CAD build for the part. Positions are in the model's coordinates, mm. Face numbers are marked on the shaded views. A direction names the side the tool comes from. Round coordinates to 2 decimals unless told otherwise and drop trailing zeros. Loops run counter-clockwise (first coordinate to the right, second up) from the corner with the lowest first, then second, coordinate; pieces in that order, holes last. Notation, with made-up numbers: (21.5, -18.5) - (62.5, -18.5) arc R28 ccw to (62.5, 0.5) - close; hole circle Ø11 at (60.25, -15.5). An arc over 180 degrees is marked (long way). One line per question, with ' | ' between items.
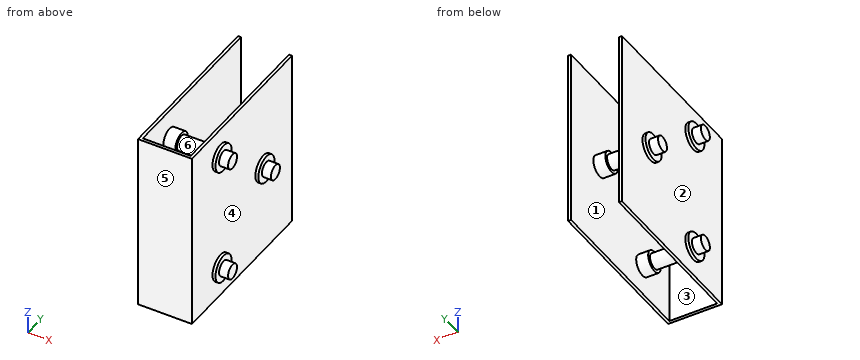
```python
from build123d import *

# Parameters (mm, degrees)
BOSS_EXTRUDE1_DEPTH      = 95.25
BOSS_EXTRUDE2_DEPTH      = 1.5875
BOSS_EXTRUDE2_DEPTH_BACK = 30.1625
SKETCH3_R                = 5.55625
SKETCH4_R                = 7.14375
BOSS_EXTRUDE3_DEPTH      = 1.5875
BOSS_EXTRUDE4_START      = 1.5875
SKETCH5_R                = 7.14375
BOSS_EXTRUDE4_DEPTH      = 1.5875
SKETCH7_W                = 12.7
SKETCH7_H                = 95.25
CUT_EXTRUDE1_DEPTH       = 131.184679518
BOSS_EXTRUDE5_DEPTH      = 6.35
BOSS_EXTRUDE5_DEPTH_BACK = 34.9377
SKETCH6_R                = 3.96875


with BuildPart() as part:
    # Sketch1 → Boss-Extrude1 (new body)
    with BuildSketch(Plane.XY):
        Polygon((-14.2875, 88.9), (-14.2875, 0), (14.2875, 0), (14.2875, 88.9), (12.7, 88.9), (12.7, 1.5875), (-12.7, 1.5875), (-12.7, 88.9), align=None)
    extrude(amount=BOSS_EXTRUDE1_DEPTH)

    # Sketch3 → Boss-Extrude2 (add, two sides: drawn at the far end of the back side and taken through both)
    with BuildSketch(Plane(origin=(14.2875, 0, 0), x_dir=(0, 0, -1), z_dir=(1, 0, 0)).offset(-BOSS_EXTRUDE2_DEPTH_BACK)):
        with Locations(Location((-47.625, 63.5, 0), (0, 0, 90))):
            Circle(SKETCH3_R)
        with Locations(Location((-79.375, 25.4, 0), (0, 0, 90))):
            Circle(SKETCH3_R)
        with Locations(Location((-15.875, 25.4, 0), (0, 0, 90))):
            Circle(SKETCH3_R)
    extrude(amount=BOSS_EXTRUDE2_DEPTH + BOSS_EXTRUDE2_DEPTH_BACK)

    # Sketch4 → Boss-Extrude3 (add)
    with BuildSketch(Plane(origin=(14.2875, 0, 0), x_dir=(0, 0, -1), z_dir=(1, 0, 0))):
        with Locations(Location((-47.625, 63.5, 0), (0, 0, 270))):
            Circle(SKETCH4_R)
        with Locations(Location((-15.875, 25.4, 0), (0, 0, 270))):
            Circle(SKETCH4_R)
        with Locations(Location((-79.375, 25.4, 0), (0, 0, 270))):
            Circle(SKETCH4_R)
    extrude(amount=BOSS_EXTRUDE3_DEPTH)

    # Sketch5 → Boss-Extrude4 (add)
    with BuildSketch(Plane.ZY.offset(14.2875).offset(BOSS_EXTRUDE4_START)):
        with Locations(Location((47.625, 63.5, 0), (0, 0, 270))):
            Circle(SKETCH5_R)
        with Locations(Location((79.375, 25.4, 0), (0, 0, 270))):
            Circle(SKETCH5_R)
        with Locations(Location((15.875, 25.4, 0), (0, 0, 270))):
            Circle(SKETCH5_R)
    extrude(amount=-BOSS_EXTRUDE4_DEPTH)

    # Sketch7 → Cut-Extrude1 (cut, through all)
    with BuildSketch(Plane(origin=(0, 1.5875, 0), x_dir=(1, 0, 0), z_dir=(0, 1, 0))):
        with Locations((0, -47.625)):
            Rectangle(SKETCH7_W, SKETCH7_H)
    extrude(amount=CUT_EXTRUDE1_DEPTH, mode=Mode.SUBTRACT)

    # Sketch6 → Boss-Extrude5 (add, two sides: drawn at the far end of the back side and taken through both)
    with BuildSketch(Plane.ZY.offset(14.2875).offset(-BOSS_EXTRUDE5_DEPTH_BACK)):
        with Locations((47.625, 63.5)):
            Circle(SKETCH6_R)
        with Locations((79.375, 25.4)):
            Circle(SKETCH6_R)
        with Locations((15.875, 25.4)):
            Circle(SKETCH6_R)
    extrude(amount=BOSS_EXTRUDE5_DEPTH + BOSS_EXTRUDE5_DEPTH_BACK)


solid = part.part
```
(1) Probe L1, parallel to X at y = 61.5, z = 80.5; L2, parallel to Y at x = -11.5, z = 33.5; L3, parallel to Y at x = -7.5, z = 80.5. List the from-to ranges inside material, lowest first.
Results found:
L1: x = -14.29 to -12.7, 12.7 to 14.29 | L2: y = 0 to 1.59 | L3: y = 0 to 1.59, 19.96 to 30.84
(2) Tool access for the marked faces 1, 2 and 3: list every direction of +Z, -Z, +X, -X, +Y, -Y with a clear straight run to the whole face (end or side of a thin tool).
Results found:
face 1: none | face 2: -X | face 3: +Z, -Z
(3) Drop flat-ended pins along their axis: P1, Ø3, axis at y = 41.5, z = 69.5, coming from the +X side; P2, Ø4, axis at x = 10, z = 35, coming from the -Y side; P3, Ø5, axis at y = 26, z = 71, coming from the +X side (3 decimals). Give the stop position or say it passes through.
Results found:
P1: stops at x = 14.29 | P2: stops at y = 0 | P3: stops at x = 15.875
(4) Cut at A-A, the plane x = -4. State how many separate pieces and enclosed holes the cut face has, then the cut area to 3 significant figures.
Results found:
separate pieces: 4 | enclosed holes: 0 | area: 300 mm²
(5) Cut at C-C, the plane z = 30. Write the cut outline in (x, y).
Results found:
outline: (-14.29, 0) - (14.29, 0) - (14.29, 88.9) - (12.7, 88.9) - (12.7, 1.59) - (-12.7, 1.59) - (-12.7, 88.9) - (-14.29, 88.9) - close
(6) Two-plate mould, pull along Y, no slides. Class the marked faces 4, 5 and 6: released by +Y, released by -Y, zero draft, split by the parting line, or undercut.
Results found:
face 4: zero draft | face 5: released by -Y | face 6: undercut
(7) Cut at B-B, the plane y = 38.5. Write the cut outline in (x, z).
Results found:
outline: (-14.29, 0) - (-12.7, 0) - (-12.7, 95.25) - (-14.29, 95.25) - close; (12.7, 0) - (14.29, 0) - (14.29, 95.25) - (12.7, 95.25) - close
